from build123d import *

# Parameters (mm, degrees)
F0_W     = 101.6
F0_H     = 127
F1_DEPTH = 6.35
F2_W     = 12.7
F2_H     = 12.7
F3_DEPTH = 152.4


with BuildPart() as f1:
    # F0 (on Front) → F1 (new body)
    with BuildSketch(Plane.XZ):
        Rectangle(F0_W, F0_H)
    extrude(amount=F1_DEPTH)

    # F2 (on face) → F3 (join)
    with BuildSketch(Plane.XZ.offset(6.35)):
        with Locations((-44.45, 57.15)):
            Rectangle(F2_W, F2_H)
        with Locations((-44.45, -57.15)):
            Rectangle(F2_W, F2_H)
        with Locations((44.45, -57.15)):
            Rectangle(F2_W, F2_H)
        with Locations((44.45, 57.15)):
            Rectangle(F2_W, F2_H)
    extrude(amount=F3_DEPTH)


solid = f1.part
Build history of the part. All positions in model axes, mm. A direction names the side the tool comes from. Coordinates: 2 decimals unless noted, no trailing zeros. Write each loop counter-clockwise with the first axis right and the second up, starting at its lowest first coordinate (ties: lowest second). Pieces come first, ordered by that corner, then holes. Notation, with made-up numbers: (24, 23) -> (82, 23) arc R22 cw to (82, 56) -> close; hole circle Ø7 at (-12.5, 40.5). An arc over 180 degrees is marked (long way). Use CSV: the item, a comma, the result in double quotes. Start each with the question number.
Q1. Cut at C-C, the plane z = 38. List the corners of the cut face in (x, y).
Q2. Pull direction X, two halves, no side cores. Call faces 1 (the flat face through (44, -158.75, 57)), 2 (the flat face through (50.8, -67, -52)), 3 (the flat face through (-1, -6.35, 1)): released by +X, released by -X, zero draft, split by the parting line, or undercut.
Q3. 3-axis set-ups, long thin cutter, end or side, ignore diameter. For faces 4 (the flat face through (44, -81, -50.8)), 5 (the flat face through (38.1, -81, 57)), 6 (the flat face through (-1, 0, 1)): which of +Z, -Z, +X, -X, +Y, -Y reach the whole face in a straight line?
Q4. Flat gauge pin, fed straight in: pin 1 Ø2 at (x, z) = (5, -35) entering from -Y. Where does the tip first touch, or does it go through?
Q5. Cut at B-B, the plane x = -19. List the corners of the cut face in (y, z), then the cut area to 3 significant figures.
Q6. Cut at A-A, the plane y = -143.5. List the corners of the cut face in (x, z).
Q7. Drill centre lines: probe 1 along X at (y, z) = (-99, 51); probe 2 along Y at (x, z) = (-27, 2). Where is each one in solid material? Low to high.
Checked values:
1,outline,"(-50.8, -6.35) -> (50.8, -6.35) -> (50.8, 0) -> (-50.8, 0) -> close"
2,face 1,"zero draft"
2,face 2,"released by +X"
2,face 3,"undercut"
3,face 4,"+X, -X, -Y"
3,face 5,"+Z, -Z, -Y"
3,face 6,"+Z, -Z, +X, -X, +Y"
4,pin 1,"stops at y = -6.35"
5,outline,"(-6.35, -63.5) -> (0, -63.5) -> (0, 63.5) -> (-6.35, 63.5) -> close"
5,area,"806 mm²"
6,outline,"(-50.8, -63.5) -> (-38.1, -63.5) -> (-38.1, -50.8) -> (-50.8, -50.8) -> close; (-50.8, 50.8) -> (-38.1, 50.8) -> (-38.1, 63.5) -> (-50.8, 63.5) -> close; (38.1, -63.5) -> (50.8, -63.5) -> (50.8, -50.8) -> (38.1, -50.8) -> close; (38.1, 50.8) -> (50.8, 50.8) -> (50.8, 63.5) -> (38.1, 63.5) -> close"
7,probe 1,"x = -50.8 to -38.1, 38.1 to 50.8"
7,probe 2,"y = -6.35 to 0"
